```python
from build123d import *

# Parameters (mm, degrees)
SKETCH1_W           = 3
SKETCH1_H           = 42.1
SKETCH1_H_2         = 4
BOSS_EXTRUDE1_DEPTH = 12
SKETCH3_W           = 45.1
SKETCH3_H           = 17.9
SKETCH3_R           = 1.5
BOSS_EXTRUDE2_DEPTH = 3
SKETCH5_W           = 17.9
SKETCH5_H           = 45.1
BOSS_EXTRUDE4_DEPTH = 4.5
CUT_EXTRUDE4_DEPTH  = 54.638254019


with BuildPart() as part:
    # Sketch1 → Boss-Extrude1 (new body)
    with BuildSketch(Plane.YZ):
        Polygon((-5.95, 3.8), (5.95, 3.8), (8.95, 3.8), (8.95, 6.8), (-8.95, 6.8), (-8.95, 3.8), align=None)
        with Locations((-7.45, -17.25)):
            Rectangle(SKETCH1_W, SKETCH1_H)
        with Locations((7.45, -17.25)):
            Rectangle(SKETCH1_W, SKETCH1_H)
        with Locations((0, -32.3)):
            Rectangle(SKETCH1_W, SKETCH1_H_2)
    extrude(amount=BOSS_EXTRUDE1_DEPTH)

    # Sketch3 → Boss-Extrude2 (add)
    with BuildSketch(Plane.ZY):
        with Locations((-15.75, 0)):
            Rectangle(SKETCH3_W, SKETCH3_H)
        Circle(SKETCH3_R, mode=Mode.SUBTRACT)
    extrude(amount=BOSS_EXTRUDE2_DEPTH)

    # Sketch5 → Boss-Extrude4 (add)
    with BuildSketch(Plane(origin=(-3, 0, 0), x_dir=(0, -1, 0), z_dir=(-1, 0, 0))):
        Polygon((-13.95, 21.583539772), (-13.95, -49.572772711), (13.95, -49.572772711), (13.95, 20.927227289), (13.95, 30.427227289), (-13.95, 30.427227289), align=None)
        with Locations((0, -15.75)):
            Rectangle(SKETCH5_W, SKETCH5_H, mode=Mode.SUBTRACT)
    extrude(amount=-BOSS_EXTRUDE4_DEPTH)

    # Sketch6 → Cut-Extrude4 (cut, symmetric)
    with BuildSketch(Plane(origin=(-3, 0, 0), x_dir=(0, -1, 0), z_dir=(-1, 0, 0))):
        with BuildLine():
            Line((-8.95, -4.430558852), (-13.95, -4.430558852))
            ThreePointArc((-13.95, -4.430558852), (-10.365862707, 0.702047669), (-8.95, 6.8))
            Line((-8.95, 6.8), (-13.95, 6.8))
            ThreePointArc((-13.95, 6.8), (-4.216827043, 16.985131712), (0, 30.427227289))
            Line((0, 30.427227289), (0, 38.207310194))
            Line((0, 38.207310194), (-27.495186948, 38.207310194))
            Line((-27.495186948, 38.207310194), (-27.495186948, -49.572772711))
            Line((-27.495186948, -49.572772711), (-5.95, -49.572772711))
            Line((-5.95, -49.572772711), (-5.95, -38.463062756))
            Line((-5.95, -38.463062756), (-13.95, -38.463062756))
            ThreePointArc((-13.95, -38.463062756), (-10.621066319, -33.1423359), (-8.95, -27.092586229))
            Line((-8.95, -27.092586229), (-13.95, -27.092586229))
            ThreePointArc((-13.95, -27.092586229), (-10.764093377, -21.676860063), (-8.95, -15.661117704))
            Line((-8.95, -15.661117704), (-13.95, -15.661117704))
            ThreePointArc((-13.95, -15.661117704), (-10.365862707, -10.528511183), (-8.95, -4.430558852))
        make_face()
    cut_extrude4 = extrude(amount=CUT_EXTRUDE4_DEPTH, both=True, mode=Mode.SUBTRACT)

    # Mirror1: Cut-Extrude4 across plane
    add(cut_extrude4.mirror(Plane.ZX), mode=Mode.SUBTRACT)


solid = part.part
```
Verification items for the finished model (mm, model axes). A direction names the side the tool comes from. Coordinates: 2 decimals unless noted, no trailing zeros. Loops run counter-clockwise (first coordinate to the right, second up) from the corner with the lowest first, then second, coordinate; pieces in that order, holes last. Notation, with made-up numbers: (12.5, 70.25) -> (29.5, 70.25) arc R14 cw to (29.5, 97.25) -> close; hole circle Ø4 at (-32, 34.5). An arc over 180 degrees is marked (long way). Answer in a Markdown table with one row per item. Add a question column.
1. Depth check by flat-ended pin: P1, Ø8, axis at x = 3, z = -8.5, coming from the -Y side; P2, Ø1.3, axis at x = 0, z = -42.5, coming from the -Y side; P3, Ø2.5, axis at y = -11.5, z = 0, coming from the +X side. Enter the tip coordinate at first touch or a pass-through.
2. Section check D-D, the plane z = 0. Enter the section's corners in (x, y).
3. Draft check along Y on faces 1 (the face through (7, -8.95, -16)), 2 (the face through (6, 0, 3.8)), 3 (the face through (-0.781, 10.402, 0.622)). Enter one of: +Y half, -Y half, draft (parallel to the pull), parting line (faces both ways), or undercut.
4. Section check A-A, the plane x = 4. Enter the section's corners in (y, z), then the cut area to 3 significant figures.
5. Section check C-C, the plane x = -2. Enter the section's corners in (y, z).
6. Access from +Z, -Z, +X, -X, +Y, -Y to the whole of each face (thin tool, end or side, straight path). Record for faces 4 (the face through (-1, -11, 6.8)), 5 (the face through (1.5, 11, -1)), 6 (the face through (-1, 11, -27.093)).
7. Material ranges on probe 1 along X at (y, z) = (1, -45.5); probe 2 along X at (y, z) = (5.5, -21.5); probe 3 along Y at (x, z) = (-0.95, 0), recorded low to high. Write a range as [from, to].
8. Section check B-B, the plane y = -10.75. Enter the section's corners in (x, z).
Derived:
| question | item | result |
|---|---|---|
| 1 | P1 | stops at y = -11.23 |
| 1 | P2 | stops at y = -5.95 |
| 1 | P3 | stops at x = 1.5 |
| 2 | outline | (-3, -10.7) -> (1.5, -10.7) -> (1.5, -8.95) -> (12, -8.95) -> (12, -5.95) -> (0, -5.95) -> (0, -1.5) -> (-3, -1.5) -> close; (-3, 1.5) -> (0, 1.5) -> (0, 5.95) -> (12, 5.95) -> (12, 8.95) -> (1.5, 8.95) -> (1.5, 10.7) -> (-3, 10.7) -> close |
| 3 | face 1 | -Y half |
| 3 | face 2 | undercut |
| 3 | face 3 | +Y half |
| 4 | outline | (-8.95, -38.3) -> (-5.95, -38.3) -> (-5.95, 3.8) -> (5.95, 3.8) -> (5.95, -38.3) -> (8.95, -38.3) -> (8.95, 6.8) -> (-8.95, 6.8) -> close; (-1.5, -34.3) -> (1.5, -34.3) -> (1.5, -30.3) -> (-1.5, -30.3) -> close |
| 4 | area | 318 mm² |
| 5 | outline | (-13.95, -38.46) -> (-5.95, -38.46) -> (-5.95, -49.57) -> (5.95, -49.57) -> (5.95, -38.46) -> (13.95, -38.46) arc R21.75 cw to (8.95, -27.09) -> (13.95, -27.09) arc R26.37 cw to (8.95, -15.66) -> (13.95, -15.66) arc R16.51 cw to (8.95, -4.43) -> (13.95, -4.43) arc R16.51 cw to (8.95, 6.8) -> (13.95, 6.8) arc R30.98 cw to (0, 30.43) arc R30.98 cw to (-13.95, 6.8) -> (-8.95, 6.8) arc R16.51 cw to (-13.95, -4.43) -> (-8.95, -4.43) arc R16.51 cw to (-13.95, -15.66) -> (-8.95, -15.66) arc R26.37 cw to (-13.95, -27.09) -> (-8.95, -27.09) arc R21.75 cw to start; hole circle Ø3 at (0, 0) |
| 6 | face 4 | +X, -X, -Y |
| 6 | face 5 | +Z, -Z, +X, +Y |
| 6 | face 6 | +X, -X, +Y |
| 7 | probe 1 | x = [-3, 1.5] |
| 7 | probe 2 | x = [-3, 0] |
| 7 | probe 3 | y = [-10.7, -1.5], [1.5, 10.7] |
| 8 | outline | (-3, -38.46) -> (1.5, -38.46) -> (1.5, -33.43) -> (-3, -33.43) -> close; (-3, -27.09) -> (1.5, -27.09) -> (1.5, -21.64) -> (-3, -21.64) -> close; (-3, -15.66) -> (1.5, -15.66) -> (1.5, -11.33) -> (-3, -11.33) -> close; (-3, -4.43) -> (1.5, -4.43) -> (1.5, -0.1) -> (-3, -0.1) -> close; (-3, 6.8) -> (1.5, 6.8) -> (1.5, 9.2) -> (-3, 9.2) -> close |
